Input: part model. Units: mm. Frame: model coordinates. A direction names the side the tool comes from. Coordinates: 2 decimals unless noted, no trailing zeros. Loops run counter-clockwise (first coordinate to the right, second up) from the corner with the lowest first, then second, coordinate; pieces in that order, holes last. Notation, with made-up numbers: M 49.5,-35.5 L 58.5,-35.5 A17 ccw 58.5,-22.5 Z; hole C 32.5,64 d1. An arc over 180 degrees is marked long. Use a Markdown table: item, result. Add a question column.
1. Draft query along X for faces 6 (the flat face through (-50.546, 73, 2)), 7 (the flat face through (-11.938, 15, 2)), 8 (the cylindrical face through (-32.1, 38.2, 2.3)). Return one class per face: +X half, -X half, draft (parallel to the pull), parting line (faces both ways), or undercut.
2. Set-up query: faces 1 (the flat face through (-4, 22.098, 2)), 2 (the flat face through (-49, 123, 2)), 3 (the cylindrical face through (-44.173, 35.174, 2.348)), 4 (the flat face through (-44.958, 15, 2)), 5 (the flat face through (-0.762, 76, 2)). Return all of +Z, -Z, +X, -X, +Y, -Y with unobstructed straight access to the full face (end or side cutting, diameter ignored); none if empty.
3. Line query: L1, parallel to Y at x = -38.1, z = 2 (3 decimals); L2, parallel to Y at x = -20.32, z = 2.7 (3 decimals); L3, parallel to Y at x = -30.5, z = 1.2 (3 decimals). Output: solid intervals per line, ascending. Write a range as [from, to].
4. Section B-B on y = 88.9. Output: boundary loops of the cut face in (x, z) (1 decimal), then the cut area to 3 significant figures.
5. Section A-A on x = -38.1. Output: boundary loops of the cut face in (y, z) (1 decimal).
6. Section C-C on z = 3.35. State how many separate pieces and enclosed holes the cut face has, then the cut area to 3 significant figures.
7. Section D-D on x = -5. Output: boundary loops of the cut face in (y, z) (1 decimal).
8. Pin query (flat end, axial travel): pin 1 (2.5 mm diameter, centred on y = 129.5, z = 2, fed in from -X); pin 2 (0.6 mm diameter, centred on x = -49, z = 2.5, fed in from +Y); pin 3 (0.9 mm diameter, centred on y = 15, z = 2, fed in from +X). Return the tip coordinate at first contact, or that it passes through.
```python
from build123d import *

# Parameters (mm, degrees)
BOSS_EXTRUDE1_DEPTH         = 4.7625
F_3_4_0_75_DIAMETER_HOLE1_D = 19.05
F_6_CLEARANCE_HOLE1_D       = 4.3053


with BuildPart() as part:
    # Sketch1 → Boss-Extrude1 (new body)
    with BuildSketch(Plane.XY):
        with BuildLine():
            Line((-0.762, 22.86), (-0.762, 130.683))
            ThreePointArc((-0.762, 130.683), (-0.985184633, 131.221815367), (-1.524, 131.445))
            Line((-1.524, 131.445), (-41.275, 131.445))
            ThreePointArc((-41.275, 131.445), (-41.813815367, 131.221815367), (-42.037, 130.683))
            Line((-42.037, 130.683), (-42.037, 128.5875))
            ThreePointArc((-42.037, 128.5875), (-43.673687307, 124.636187307), (-47.625, 122.9995))
            Line((-47.625, 122.9995), (-49.784, 122.9995))
            ThreePointArc((-49.784, 122.9995), (-50.322815367, 122.776315367), (-50.546, 122.2375))
            Line((-50.546, 122.2375), (-50.546, 22.814114212))
            ThreePointArc((-50.546, 22.814114212), (-50.354228586, 22.308660594), (-49.87544, 22.057620507))
            ThreePointArc((-49.87544, 22.057620507), (-46.364323705, 20.216659866), (-44.958, 16.51))
            Line((-44.958, 16.51), (-44.958, 13.462))
            ThreePointArc((-44.958, 13.462), (-44.734815367, 12.923184633), (-44.196, 12.7))
            Line((-44.196, 12.7), (-12.7, 12.7))
            ThreePointArc((-12.7, 12.7), (-12.161184633, 12.923184633), (-11.938, 13.462))
            Line((-11.938, 13.462), (-11.938, 16.51))
            ThreePointArc((-11.938, 16.51), (-10.301312693, 20.461312693), (-6.35, 22.098))
            Line((-6.35, 22.098), (-1.524, 22.098))
            ThreePointArc((-1.524, 22.098), (-0.985184633, 22.321184633), (-0.762, 22.86))
        make_face()
    extrude(amount=BOSS_EXTRUDE1_DEPTH)

    # 3/4 (0.75) Diameter Hole1 (through all)
    with Locations(Plane.XY.offset(4.7625)):
        with Locations((-38.1, 88.9), (-11.684, 88.9), (-26.9875, 30.1625)):
            Hole(F_3_4_0_75_DIAMETER_HOLE1_D / 2)

    # #6 Clearance Hole1 (through all)
    with Locations(Plane.XY.offset(4.7625)):
        with Locations((-20.32, 120.65), (-43.18, 37.084)):
            Hole(F_6_CLEARANCE_HOLE1_D / 2)


solid = part.part
```
Answers below:
| question | item | result |
|---|---|---|
| 1 | face 6 | -X half |
| 1 | face 7 | +X half |
| 1 | face 8 | undercut |
| 2 | face 1 | +Z, -Z, +X, -Y |
| 2 | face 2 | +Z, -Z, -X, +Y |
| 2 | face 3 | +Z, -Z |
| 2 | face 4 | +Z, -Z, -X, -Y |
| 2 | face 5 | +Z, -Z, +X, +Y, -Y |
| 3 | L1 | y = [12.7, 79.375], [98.425, 131.445] |
| 3 | L2 | y = [12.7, 23.36], [36.965, 84.882], [92.918, 118.497], [122.803, 131.445] |
| 3 | L3 | y = [12.7, 21.309], [39.016, 83.158], [94.642, 131.445] |
| 4 | outline | M -50.5,0 L -47.6,0 L -47.6,4.8 L -50.5,4.8 Z; M -28.6,0 L -21.2,0 L -21.2,4.8 L -28.6,4.8 Z; M -2.2,0 L -0.8,0 L -0.8,4.8 L -2.2,4.8 Z |
| 4 | area | 55.6 mm² |
| 5 | outline | M 12.7,0 L 79.4,0 L 79.4,4.8 L 12.7,4.8 Z; M 98.4,0 L 131.4,0 L 131.4,4.8 L 98.4,4.8 Z |
| 6 | separate pieces | 1 |
| 6 | enclosed holes | 5 |
| 6 | area | 4,820 mm² |
| 7 | outline | M 22.1,0 L 82.1,0 L 82.1,4.8 L 22.1,4.8 Z; M 95.7,0 L 131.4,0 L 131.4,4.8 L 95.7,4.8 Z |
| 8 | pin 1 | stops at x = -42.05 |
| 8 | pin 2 | stops at y = 123 |
| 8 | pin 3 | stops at x = -11.94 |
